Autodesk Inventor part; units mm, degrees
ref_plane "body_to_dummy_XY" through (0, 0, 0) normal (0, -1, 0) x (1, 0, 0)
ref_plane "body_to_dummy_YZ" through (0, 0, 0) normal (1, 0, 0) x (0, 0, 1)
ref_plane "body_to_dummy_ZX" through (0, 0, 0) normal (0, 0, 1) x (0, -1, 0)
sketch "Sketch_1" plane through (0, 0, 0) normal (0, 1, 0) x (1, 0, 0)
  line L0 (-2.54, 1.27) -> (-2.54, -1.27)
  line L1 (-2.54, -1.27) -> (2.54, -1.27)
  line L2 (2.54, -1.27) -> (2.54, 1.27)
  line L3 (2.54, 1.27) -> (-2.54, 1.27)
extrude "Extrusion1" add sketch "Sketch_1" along normal blind 6.096
sketch "Sketch_2" plane through (0, 5.461, 0) normal (0, 1, 0) x (1, 0, 0)
  line L0 (-2.794, 2.54) -> (-2.794, -2.54)
  line L1 (-2.794, -2.54) -> (2.794, -2.54)
  line L2 (2.794, -2.54) -> (2.794, 2.54)
  line L3 (2.794, 2.54) -> (-2.794, 2.54)
  line L4 (-2.286, 1.016) -> (-2.286, -1.016)
  line L5 (-2.286, -1.016) -> (2.286, -1.016)
  line L6 (2.286, -1.016) -> (2.286, 1.016)
  line L7 (2.286, 1.016) -> (-2.286, 1.016)
extrude "Extrusion2" cut sketch "Sketch_2" against normal blind 0.508
sketch "Sketch_3" plane through (0, 6.096, 0) normal (0, 1, 0) x (1, 0, 0)
  line L0 (-0.762, 1.27) -> (-0.762, -1.27)
  line L1 (-0.762, -1.27) -> (0.762, -1.27)
  line L2 (0.762, -1.27) -> (0.762, 1.27)
  line L3 (0.762, 1.27) -> (-0.762, 1.27)
extrude "Extrusion3" cut sketch "Sketch_3" against normal blind 2.54
sketch "Sketch_4" plane through (0, 6.096, 0) normal (0, 1, 0) x (1, 0, 0)
  line L0 (-1.778, 0.4445) -> (-1.778, -0.4445)
  line L1 (-1.778, -0.4445) -> (1.778, -0.4445)
  line L2 (1.778, -0.4445) -> (1.778, 0.4445)
  line L3 (1.778, 0.4445) -> (-1.778, 0.4445)
extrude "Extrusion4" cut sketch "Sketch_4" against normal blind 6.096
sketch "Sketch_5" plane through (0, 5.7912, 0) normal (0, 1, 0) x (1, 0, 0)
  line L0 (-2.032, 0.5969) -> (-2.032, -0.5969)
  line L1 (-2.032, -0.5969) -> (2.032, -0.5969)
  line L2 (2.032, -0.5969) -> (2.032, 0.5969)
  line L3 (2.032, 0.5969) -> (-2.032, 0.5969)
extrude "Extrusion5" cut sketch "Sketch_5" against normal blind 6.096
sketch "Sketch_8" plane through (0, 0, 0) normal (0, 1, 0) x (-1, 0, 0)
  line L0 (0.762, -0.6477) -> (0.762, 0.6477)
  line L1 (0.762, 0.6477) -> (-0.762, 0.6477)
  line L2 (-0.762, 0.6477) -> (-0.762, -0.6477)
  line L3 (-0.762, -0.6477) -> (0.762, -0.6477)
extrude "Extrusion6" cut sketch "Sketch_8" along normal blind 3.556
sketch "Sketch_6" plane through (0, 0, 0) normal (1, 0, 0) x (0, 1, 0)
  line L0 (3.0093, 0.2159) -> (2.2752, -0.6477)
  line L1 (2.2752, -0.6477) -> (6.096, -0.6477)
  line L2 (6.096, -0.6477) -> (6.096, 0.2159)
  line L3 (6.096, 0.2159) -> (3.0093, 0.2159)
extrude "Extrusion7" add sketch "Sketch_6" along normal mid plane 1.27
ref_plane "body_to_dummy_XY" through (0, 0, 0) normal (0, -1, 0) x (1, 0, 0)
ref_plane "body_to_dummy_YZ" through (0, 0, 0) normal (1, 0, 0) x (0, 0, 1)
ref_plane "body_to_dummy_ZX" through (0, 0, 0) normal (0, 0, 1) x (0, -1, 0)
properties part number "SNT-100-BK_body"
Read the model definition and answer for the solid it produces. Units are mm, in the model's axes. A direction names the side the tool comes from. Coordinates: 2 decimals unless noted, no trailing zeros. Loops run counter-clockwise (first coordinate to the right, second up) from the corner with the lowest first, then second, coordinate; pieces in that order, holes last. Notation, with made-up numbers: (-29.75, 45.25) - (-18.75, 45.25) arc R5 ccw to (-18.75, 52.25) - close; hole circle Ø10 at (40, 73.25). An arc over 180 degrees is marked (long way). Answer in a Markdown table with one row per item.
Q1. Find section C-C on z = -1.1. Write down the section's boundary in (x, y), plus the area to 3 significant figures.
Here are the results:
| item | result |
|---|---|
| outline | (-2.54, 0) - (2.54, 0) - (2.54, 4.95) - (0.76, 4.95) - (0.76, 3.56) - (-0.76, 3.56) - (-0.76, 4.95) - (-2.54, 4.95) - close; (-2.54, 5.46) - (-0.76, 5.46) - (-0.76, 6.1) - (-2.54, 6.1) - close; (0.76, 5.46) - (2.54, 5.46) - (2.54, 6.1) - (0.76, 6.1) - close |
| area | 25.3 mm^2 |
Q2. Find section B-B on y = 3.75. Write down the section's boundary in (x, z) (3 decimals), plus the area to 3 significant figures.
Here are the results:
| item | result |
|---|---|
| outline | (-2.54, -1.27) - (-0.762, -1.27) - (-0.762, -0.597) - (-2.032, -0.597) - (-2.032, 0.597) - (-0.762, 0.597) - (-0.762, 1.27) - (-2.54, 1.27) - close; (-0.635, -0.648) - (0.635, -0.648) - (0.635, 0.216) - (-0.635, 0.216) - close; (0.762, -1.27) - (2.54, -1.27) - (2.54, 1.27) - (0.762, 1.27) - (0.762, 0.597) - (2.032, 0.597) - (2.032, -0.597) - (0.762, -0.597) - close |
| area | 7.10 mm^2 |
Q3. For faces 1 (the flat face through (0, 1, -0.648)), 2 (the flat face through (0, 5, -0.648)), 3 (the flat face through (0, 2, 0.648)), determine the directions among +Z, -Z, +X, -X, +Y, -Y from which every point of the face is accessible in a straight line to the end or side of a thin tool.
Here are the results:
| item | result |
|---|---|
| face 1 | -Y |
| face 2 | -Z, +Y |
| face 3 | +Y, -Y |
Q4. Straight lines are drawn through the part: line 1 along Y through (x, z) = (2.3, -1.05); line 2 along X through (y, z) = (3, -0.25) (3 decimals); line 3 along Z through (x, y) = (-1.45, 1.5). For each, find the intervals that lie inside material, in ascending order. Write a range as [from, to].
Here are the results:
| item | result |
|---|---|
| line 1 | y = [0, 4.95], [5.46, 6.1] |
| line 2 | x = [-2.54, -2.032], [-0.635, 0.635], [2.032, 2.54] |
| line 3 | z = [-1.27, -0.6], [0.6, 1.27] |
Q5. Given P1, Ø0.7, axis at x = 0, z = 1, coming from the +Y side, flat-ended and moving along its own axis, determine where the tip first touches the part or whether it passes through.
Here are the results:
| item | result |
|---|---|
| P1 | stops at y = 3.56 |
Q6. Find section A-A on x = 1.45. Write down the section's boundary in (y, z).
Here are the results:
| item | result |
|---|---|
| outline | (0, -1.27) - (4.95, -1.27) - (4.95, -1.02) - (5.46, -1.02) - (5.46, -1.27) - (6.1, -1.27) - (6.1, -0.44) - (5.79, -0.44) - (5.79, -0.6) - (0, -0.6) - close; (0, 0.6) - (5.79, 0.6) - (5.79, 0.44) - (6.1, 0.44) - (6.1, 1.27) - (5.46, 1.27) - (5.46, 1.02) - (4.95, 1.02) - (4.95, 1.27) - (0, 1.27) - close |
Q7. Find section D-D on y = 0.75. Write down the section's boundary in (x, z), plus the area to 3 significant figures.
Here are the results:
| item | result |
|---|---|
| outline | (-2.54, -1.27) - (2.54, -1.27) - (2.54, 1.27) - (-2.54, 1.27) - close; hole (-2.03, -0.6) - (-0.76, -0.6) - (-0.76, -0.65) - (0.76, -0.65) - (0.76, -0.6) - (2.03, -0.6) - (2.03, 0.6) - (0.76, 0.6) - (0.76, 0.65) - (-0.76, 0.65) - (-0.76, 0.6) - (-2.03, 0.6) - close |
| area | 7.90 mm^2 |
Q8. The mould has two halves that part along X. Classify faces 4 (the flat face through (0, 6.096, 0)), 5 (the flat face through (0.762, 4, 1)): pulls with the +X half, pulls with the -X half, needs draft (parallel to the pull), parting line crosses it, or undercut.
Here are the results:
| item | result |
|---|---|
| face 4 | needs draft |
| face 5 | undercut |
